For this review, use the dimensioned drawing (mm, ordinates from the lowest corner) and the shaded views. A direction names the side the tool comes from. Round coordinates to 2 decimals unless told otherwise and drop trailing zeros. Order: outer loops, then holes, each group sorted by start corner. A loop starts at its lowest first (then second) coordinate and runs counter-clockwise, first axis right, second up. Notation, with made-up numbers: (34, 58.5) -> (81, 58.5) arc R13 cw to (81, 77.5) -> close; hole circle Ø9 at (-35.5, 12). An arc over 180 degrees is marked (long way). Use a Markdown table: item, result. Add a question column.
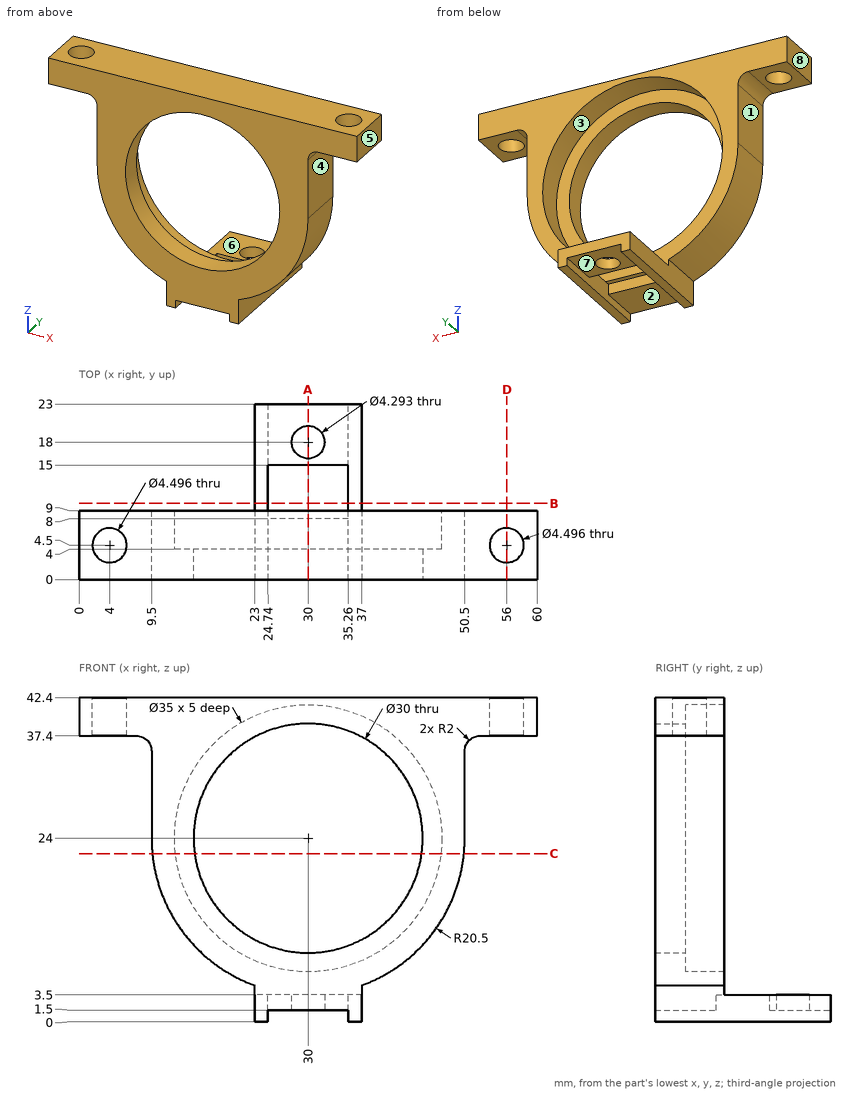
Q1. Insertion check: pin 1 (11.5 mm diameter, centred on x = 39, z = 28, fed in from +Y); pin 2 (3.5 mm diameter, centred on x = 30, y = 18, fed in from +Z); pin 3 (7 mm diameter, centred on y = 2.5, z = 29.5, fed in from -X); pin 4 (4 mm diameter, centred on x = 57.5, y = 5, fed in from -Z). Each pin has a flat end and moves straight along its axis. Give the tip position at first contact, or say it passes through.
Q2. Machinability: for the marked faces 1, 2, 3, 4 and 5, which of the approach directions +Z, -Z, +X, -X, +Y, -Y give a long, thin tool a straight path to every point of the face, cutting with its end or side? Answer none if there is none.
Q3. Add section C-C (z = 22). Write out the cut boundary in (x, y) (1 decimal).
Q4. Add section B-B (y = 10). Write out the cut boundary in (x, z).
Q5. Wall thickness on line 1 (Y direction, x = 30, z = 2); line 2 (Z direction, x = 30, y = 2.75); line 3 (Y direction, x = 4, z = 38.7): over which ranges is each line inside the solid? List them lowest first. Write a range as [from, to].
Q6. Add section A-A (x = 30). Write out the cut boundary in (y, z).
Q7. Add section D-D (x = 56). Write out the cut boundary in (y, z).
Q8. Mouldability with a two-part tool opening along X and no side actions: class the marked faces 6, 7 and 8 as pulls with the +X half, pulls with the -X half, needs draft (parallel to the pull), parting line crosses it, or undercut.
Report:
| question | item | result |
|---|---|---|
| 1 | pin 1 | stops at y = 4 |
| 1 | pin 2 | passes through |
| 1 | pin 3 | stops at x = 9.5 |
| 1 | pin 4 | stops at z = 37.4 |
| 2 | face 1 | -Z, -X, +Y, -Y |
| 2 | face 2 | -Z, +Y, -Y |
| 2 | face 3 | +Y |
| 2 | face 4 | -Z, +X, +Y, -Y |
| 2 | face 5 | +Z, -Z, +X, +Y, -Y |
| 3 | outline | (9.6, 0) -> (15.1, 0) -> (15.1, 4) -> (12.6, 4) -> (12.6, 9) -> (9.6, 9) -> close; (44.9, 0) -> (50.4, 0) -> (50.4, 9) -> (47.4, 9) -> (47.4, 4) -> (44.9, 4) -> close |
| 4 | outline | (23, 0) -> (24.74, 0) -> (24.74, 3.5) -> (23, 3.5) -> close; (35.26, 0) -> (37, 0) -> (37, 3.5) -> (35.26, 3.5) -> close |
| 5 | line 1 | y = [0, 8], [15, 15.85], [20.15, 23] |
| 5 | line 2 | z = [1.5, 9], [39, 42.4] |
| 5 | line 3 | y = [0, 2.25], [6.75, 9] |
| 6 | outline | (0, 1.5) -> (8, 1.5) -> (8, 3.5) -> (9, 3.5) -> (9, 6.5) -> (4, 6.5) -> (4, 9) -> (0, 9) -> close; (0, 39) -> (4, 39) -> (4, 41.5) -> (9, 41.5) -> (9, 42.4) -> (0, 42.4) -> close; (15, 1.5) -> (15.85, 1.5) -> (15.85, 3.5) -> (15, 3.5) -> close; (20.15, 1.5) -> (23, 1.5) -> (23, 3.5) -> (20.15, 3.5) -> close |
| 7 | outline | (0, 37.4) -> (2.25, 37.4) -> (2.25, 42.4) -> (0, 42.4) -> close; (6.75, 37.4) -> (9, 37.4) -> (9, 42.4) -> (6.75, 42.4) -> close |
| 8 | face 6 | needs draft |
| 8 | face 7 | undercut |
| 8 | face 8 | pulls with the -X half |
